Check sheet for the modelled part. Datum: model origin and axes. Units: mm. A direction names the side the tool comes from. Round coordinates to 2 decimals unless told otherwise and drop trailing zeros. Write each loop counter-clockwise with the first axis right and the second up, starting at its lowest first coordinate (ties: lowest second). Pieces come first, ordered by that corner, then holes. Notation, with made-up numbers: (68, 56) - (102, 56) arc R21 ccw to (102, 60) - close; hole circle Ø1 at (66, -12.5). An arc over 180 degrees is marked (long way). Use one line per item in the form item = value. Start each with the question number.
1) Scan lines: probe 1 along Z at (x, y) = (-1.5, -5); probe 2 along X at (y, z) = (-5.75, 16.5); probe 3 along Z at (x, y) = (5.25, 4.25). Record each from-to range of solid material in increasing order.
2) Gauge pin test, flat ends, axial feed: P1, Ø3, axis at y = 2, z = 31.5, coming from the +X side; P2, Ø1, axis at x = -4, y = 6, coming from the +Z side; P3, Ø8, axis at x = 0.5, y = 5.5, coming from the +Z side. Record the tip position at first contact, or that the pin passes through.
3) Section check C-C (z = 41). Record the boundary of the cut face in (x, y), then the cut area to 3 significant figures.
4) Section check B-B (z = 36). Record the boundary of the cut face in (x, y), then the cut area to 3 significant figures.
5) Set-up check for faces 1 (the face through (-3.746, 0.165, 37.708)), 2 (the face through (0, 0.75, 44)), 3 (the face through (0, -0.75, 44)): record each of +Z, -Z, +X, -X, +Y, -Y from which the full face is reachable in a straight line by a thin tool's end or side.
6) Section check A-A (z = 3). Record the boundary of the cut face in (x, y) (3 decimals).
from build123d import *

# Parameters (mm, degrees)
F1_DEPTH  = 20
F2_R      = 6
F3_DEPTH  = 15
F5_DEPTH  = 15
F6_COUNT  = 55
F8_R      = 3.75
F9_DEPTH  = 10
F11_DEPTH = 25


with BuildPart() as f1:
    # F0 (on Top) → F1 (new body)
    with BuildSketch(Plane.XY):
        Polygon((6.875, -3.969283), (6.875, 3.969283), (0, 7.938566), (-6.875, 3.969283), (-6.875, -3.969283), (0, -7.938566), align=None)
    extrude(amount=F1_DEPTH)

    # F2 (on face) → F3 (join)
    with BuildSketch(Plane.XY.offset(20)):
        Circle(F2_R)
    extrude(amount=F3_DEPTH)


with BuildPart() as f5:
    # F4 (on face) → F5 (new body, through all)
    with BuildSketch(Plane.XY.offset(35)):
        with BuildLine():
            ThreePointArc((0.365715, 5.988844), (0, 6), (-0.365715, 5.988844))
            Line((-0.365715, 5.988844), (0, 5.647886))
            Line((0, 5.647886), (0.365715, 5.988844))
        make_face()
    extrude(amount=-F5_DEPTH)


with BuildPart() as f6_1:
    # F6: instance of F5
    add(f5.part.rotate(Axis((0, 0, 35), (0, 0, -1)), 1 * 360 / F6_COUNT))


with BuildPart() as f6_2:
    # F6: instance of F5
    add(f5.part.rotate(Axis((0, 0, 35), (0, 0, -1)), 2 * 360 / F6_COUNT))


with BuildPart() as f6_3:
    # F6: instance of F5
    add(f5.part.rotate(Axis((0, 0, 35), (0, 0, -1)), 3 * 360 / F6_COUNT))


with BuildPart() as f6_4:
    # F6: instance of F5
    add(f5.part.rotate(Axis((0, 0, 35), (0, 0, -1)), 4 * 360 / F6_COUNT))


with BuildPart() as f6_5:
    # F6: instance of F5
    add(f5.part.rotate(Axis((0, 0, 35), (0, 0, -1)), 5 * 360 / F6_COUNT))


with BuildPart() as f6_6:
    # F6: instance of F5
    add(f5.part.rotate(Axis((0, 0, 35), (0, 0, -1)), 6 * 360 / F6_COUNT))


with BuildPart() as f6_7:
    # F6: instance of F5
    add(f5.part.rotate(Axis((0, 0, 35), (0, 0, -1)), 7 * 360 / F6_COUNT))


with BuildPart() as f6_8:
    # F6: instance of F5
    add(f5.part.rotate(Axis((0, 0, 35), (0, 0, -1)), 8 * 360 / F6_COUNT))


with BuildPart() as f6_9:
    # F6: instance of F5
    add(f5.part.rotate(Axis((0, 0, 35), (0, 0, -1)), 9 * 360 / F6_COUNT))


with BuildPart() as f6_10:
    # F6: instance of F5
    add(f5.part.rotate(Axis((0, 0, 35), (0, 0, -1)), 10 * 360 / F6_COUNT))


with BuildPart() as f6_11:
    # F6: instance of F5
    add(f5.part.rotate(Axis((0, 0, 35), (0, 0, -1)), 11 * 360 / F6_COUNT))


with BuildPart() as f6_12:
    # F6: instance of F5
    add(f5.part.rotate(Axis((0, 0, 35), (0, 0, -1)), 12 * 360 / F6_COUNT))


with BuildPart() as f6_13:
    # F6: instance of F5
    add(f5.part.rotate(Axis((0, 0, 35), (0, 0, -1)), 13 * 360 / F6_COUNT))


with BuildPart() as f6_14:
    # F6: instance of F5
    add(f5.part.rotate(Axis((0, 0, 35), (0, 0, -1)), 14 * 360 / F6_COUNT))


with BuildPart() as f6_15:
    # F6: instance of F5
    add(f5.part.rotate(Axis((0, 0, 35), (0, 0, -1)), 15 * 360 / F6_COUNT))


with BuildPart() as f6_16:
    # F6: instance of F5
    add(f5.part.rotate(Axis((0, 0, 35), (0, 0, -1)), 16 * 360 / F6_COUNT))


with BuildPart() as f6_17:
    # F6: instance of F5
    add(f5.part.rotate(Axis((0, 0, 35), (0, 0, -1)), 17 * 360 / F6_COUNT))


with BuildPart() as f6_18:
    # F6: instance of F5
    add(f5.part.rotate(Axis((0, 0, 35), (0, 0, -1)), 18 * 360 / F6_COUNT))


with BuildPart() as f6_19:
    # F6: instance of F5
    add(f5.part.rotate(Axis((0, 0, 35), (0, 0, -1)), 19 * 360 / F6_COUNT))


with BuildPart() as f6_20:
    # F6: instance of F5
    add(f5.part.rotate(Axis((0, 0, 35), (0, 0, -1)), 20 * 360 / F6_COUNT))


with BuildPart() as f6_21:
    # F6: instance of F5
    add(f5.part.rotate(Axis((0, 0, 35), (0, 0, -1)), 21 * 360 / F6_COUNT))


with BuildPart() as f6_22:
    # F6: instance of F5
    add(f5.part.rotate(Axis((0, 0, 35), (0, 0, -1)), 22 * 360 / F6_COUNT))


with BuildPart() as f6_23:
    # F6: instance of F5
    add(f5.part.rotate(Axis((0, 0, 35), (0, 0, -1)), 23 * 360 / F6_COUNT))


with BuildPart() as f6_24:
    # F6: instance of F5
    add(f5.part.rotate(Axis((0, 0, 35), (0, 0, -1)), 24 * 360 / F6_COUNT))


with BuildPart() as f6_25:
    # F6: instance of F5
    add(f5.part.rotate(Axis((0, 0, 35), (0, 0, -1)), 25 * 360 / F6_COUNT))


with BuildPart() as f6_26:
    # F6: instance of F5
    add(f5.part.rotate(Axis((0, 0, 35), (0, 0, -1)), 26 * 360 / F6_COUNT))


with BuildPart() as f6_27:
    # F6: instance of F5
    add(f5.part.rotate(Axis((0, 0, 35), (0, 0, -1)), 27 * 360 / F6_COUNT))


with BuildPart() as f6_28:
    # F6: instance of F5
    add(f5.part.rotate(Axis((0, 0, 35), (0, 0, -1)), 28 * 360 / F6_COUNT))


with BuildPart() as f6_29:
    # F6: instance of F5
    add(f5.part.rotate(Axis((0, 0, 35), (0, 0, -1)), 29 * 360 / F6_COUNT))


with BuildPart() as f6_30:
    # F6: instance of F5
    add(f5.part.rotate(Axis((0, 0, 35), (0, 0, -1)), 30 * 360 / F6_COUNT))


with BuildPart() as f6_31:
    # F6: instance of F5
    add(f5.part.rotate(Axis((0, 0, 35), (0, 0, -1)), 31 * 360 / F6_COUNT))


with BuildPart() as f6_32:
    # F6: instance of F5
    add(f5.part.rotate(Axis((0, 0, 35), (0, 0, -1)), 32 * 360 / F6_COUNT))


with BuildPart() as f6_33:
    # F6: instance of F5
    add(f5.part.rotate(Axis((0, 0, 35), (0, 0, -1)), 33 * 360 / F6_COUNT))


with BuildPart() as f6_34:
    # F6: instance of F5
    add(f5.part.rotate(Axis((0, 0, 35), (0, 0, -1)), 34 * 360 / F6_COUNT))


with BuildPart() as f6_35:
    # F6: instance of F5
    add(f5.part.rotate(Axis((0, 0, 35), (0, 0, -1)), 35 * 360 / F6_COUNT))


with BuildPart() as f6_36:
    # F6: instance of F5
    add(f5.part.rotate(Axis((0, 0, 35), (0, 0, -1)), 36 * 360 / F6_COUNT))


with BuildPart() as f6_37:
    # F6: instance of F5
    add(f5.part.rotate(Axis((0, 0, 35), (0, 0, -1)), 37 * 360 / F6_COUNT))


with BuildPart() as f6_38:
    # F6: instance of F5
    add(f5.part.rotate(Axis((0, 0, 35), (0, 0, -1)), 38 * 360 / F6_COUNT))


with BuildPart() as f6_39:
    # F6: instance of F5
    add(f5.part.rotate(Axis((0, 0, 35), (0, 0, -1)), 39 * 360 / F6_COUNT))


with BuildPart() as f6_40:
    # F6: instance of F5
    add(f5.part.rotate(Axis((0, 0, 35), (0, 0, -1)), 40 * 360 / F6_COUNT))


with BuildPart() as f6_41:
    # F6: instance of F5
    add(f5.part.rotate(Axis((0, 0, 35), (0, 0, -1)), 41 * 360 / F6_COUNT))


with BuildPart() as f6_42:
    # F6: instance of F5
    add(f5.part.rotate(Axis((0, 0, 35), (0, 0, -1)), 42 * 360 / F6_COUNT))


with BuildPart() as f6_43:
    # F6: instance of F5
    add(f5.part.rotate(Axis((0, 0, 35), (0, 0, -1)), 43 * 360 / F6_COUNT))


with BuildPart() as f6_44:
    # F6: instance of F5
    add(f5.part.rotate(Axis((0, 0, 35), (0, 0, -1)), 44 * 360 / F6_COUNT))


with BuildPart() as f6_45:
    # F6: instance of F5
    add(f5.part.rotate(Axis((0, 0, 35), (0, 0, -1)), 45 * 360 / F6_COUNT))


with BuildPart() as f6_46:
    # F6: instance of F5
    add(f5.part.rotate(Axis((0, 0, 35), (0, 0, -1)), 46 * 360 / F6_COUNT))


with BuildPart() as f6_47:
    # F6: instance of F5
    add(f5.part.rotate(Axis((0, 0, 35), (0, 0, -1)), 47 * 360 / F6_COUNT))


with BuildPart() as f6_48:
    # F6: instance of F5
    add(f5.part.rotate(Axis((0, 0, 35), (0, 0, -1)), 48 * 360 / F6_COUNT))


with BuildPart() as f6_49:
    # F6: instance of F5
    add(f5.part.rotate(Axis((0, 0, 35), (0, 0, -1)), 49 * 360 / F6_COUNT))


with BuildPart() as f6_50:
    # F6: instance of F5
    add(f5.part.rotate(Axis((0, 0, 35), (0, 0, -1)), 50 * 360 / F6_COUNT))


with BuildPart() as f6_51:
    # F6: instance of F5
    add(f5.part.rotate(Axis((0, 0, 35), (0, 0, -1)), 51 * 360 / F6_COUNT))


with BuildPart() as f6_52:
    # F6: instance of F5
    add(f5.part.rotate(Axis((0, 0, 35), (0, 0, -1)), 52 * 360 / F6_COUNT))


with BuildPart() as f6_53:
    # F6: instance of F5
    add(f5.part.rotate(Axis((0, 0, 35), (0, 0, -1)), 53 * 360 / F6_COUNT))


with BuildPart() as f6_54:
    # F6: instance of F5
    add(f5.part.rotate(Axis((0, 0, 35), (0, 0, -1)), 54 * 360 / F6_COUNT))


with BuildPart() as f1_1:
    add(f1.part)

    # F7: cut F6_6, F6_8, F6_10, F6_7, F6_1, F6_4, F6_5, F6_3, F6_2, F5, F6_9, F6_11, F6_12, F6_13, F6_14, F6_15, F6_16, F6_17, F6_18, F6_19, F6_20, F6_21, F6_22, F6_23, F6_24, F6_25, F6_26, F6_27, F6_28, F6_29, F6_30, F6_31, F6_32, F6_33, F6_34, F6_35, F6_36, F6_37, F6_38, F6_39, F6_40, F6_41, F6_42, F6_43, F6_44, F6_45, F6_46, F6_47, F6_48, F6_49, F6_50, F6_51, F6_52, F6_53, F6_54
    add(f6_6.part, mode=Mode.SUBTRACT)
    add(f6_8.part, mode=Mode.SUBTRACT)
    add(f6_10.part, mode=Mode.SUBTRACT)
    add(f6_7.part, mode=Mode.SUBTRACT)
    add(f6_1.part, mode=Mode.SUBTRACT)
    add(f6_4.part, mode=Mode.SUBTRACT)
    add(f6_5.part, mode=Mode.SUBTRACT)
    add(f6_3.part, mode=Mode.SUBTRACT)
    add(f6_2.part, mode=Mode.SUBTRACT)
    add(f5.part, mode=Mode.SUBTRACT)
    add(f6_9.part, mode=Mode.SUBTRACT)
    add(f6_11.part, mode=Mode.SUBTRACT)
    add(f6_12.part, mode=Mode.SUBTRACT)
    add(f6_13.part, mode=Mode.SUBTRACT)
    add(f6_14.part, mode=Mode.SUBTRACT)
    add(f6_15.part, mode=Mode.SUBTRACT)
    add(f6_16.part, mode=Mode.SUBTRACT)
    add(f6_17.part, mode=Mode.SUBTRACT)
    add(f6_18.part, mode=Mode.SUBTRACT)
    add(f6_19.part, mode=Mode.SUBTRACT)
    add(f6_20.part, mode=Mode.SUBTRACT)
    add(f6_21.part, mode=Mode.SUBTRACT)
    add(f6_22.part, mode=Mode.SUBTRACT)
    add(f6_23.part, mode=Mode.SUBTRACT)
    add(f6_24.part, mode=Mode.SUBTRACT)
    add(f6_25.part, mode=Mode.SUBTRACT)
    add(f6_26.part, mode=Mode.SUBTRACT)
    add(f6_27.part, mode=Mode.SUBTRACT)
    add(f6_28.part, mode=Mode.SUBTRACT)
    add(f6_29.part, mode=Mode.SUBTRACT)
    add(f6_30.part, mode=Mode.SUBTRACT)
    add(f6_31.part, mode=Mode.SUBTRACT)
    add(f6_32.part, mode=Mode.SUBTRACT)
    add(f6_33.part, mode=Mode.SUBTRACT)
    add(f6_34.part, mode=Mode.SUBTRACT)
    add(f6_35.part, mode=Mode.SUBTRACT)
    add(f6_36.part, mode=Mode.SUBTRACT)
    add(f6_37.part, mode=Mode.SUBTRACT)
    add(f6_38.part, mode=Mode.SUBTRACT)
    add(f6_39.part, mode=Mode.SUBTRACT)
    add(f6_40.part, mode=Mode.SUBTRACT)
    add(f6_41.part, mode=Mode.SUBTRACT)
    add(f6_42.part, mode=Mode.SUBTRACT)
    add(f6_43.part, mode=Mode.SUBTRACT)
    add(f6_44.part, mode=Mode.SUBTRACT)
    add(f6_45.part, mode=Mode.SUBTRACT)
    add(f6_46.part, mode=Mode.SUBTRACT)
    add(f6_47.part, mode=Mode.SUBTRACT)
    add(f6_48.part, mode=Mode.SUBTRACT)
    add(f6_49.part, mode=Mode.SUBTRACT)
    add(f6_50.part, mode=Mode.SUBTRACT)
    add(f6_51.part, mode=Mode.SUBTRACT)
    add(f6_52.part, mode=Mode.SUBTRACT)
    add(f6_53.part, mode=Mode.SUBTRACT)
    add(f6_54.part, mode=Mode.SUBTRACT)

    # F8 (on face) → F9 (join)
    with BuildSketch(Plane.XY.offset(35)):
        Circle(F8_R)
    extrude(amount=F9_DEPTH)

    # F10 (on face) → F11 (cut)
    with BuildSketch(Plane(origin=(-6.875, 0, 0), x_dir=(0, -1, 0), z_dir=(-1, 0, 0))):
        with BuildLine():
            Line((-0.75, 49.5), (-0.75, 50))
            Line((-0.75, 50), (-4.25, 50))
            Line((-4.25, 50), (-4.25, 36.5))
            ThreePointArc((-4.25, 36.5), (-1.673762, 39.586881), (-0.75, 43.5))
            Line((-0.75, 43.5), (-0.75, 49.5))
        make_face()
        with BuildLine():
            Line((0.75, 50), (0.75, 43.5))
            ThreePointArc((0.75, 43.5), (1.673762, 39.586881), (4.25, 36.5))
            Line((4.25, 36.5), (4.25, 50))
            Line((4.25, 50), (0.75, 50))
        make_face()
    extrude(amount=-F11_DEPTH, mode=Mode.SUBTRACT)


solid = f1_1.part
Results are:
q1.probe_1 = 0 to 35
q1.probe_2 = -3.79 to 3.79
q1.probe_3 = 0 to 20
q2.P1 = 5.91
q2.P2 = 20
q2.P3 = 39.96
q3.outline = (-3.58, -1.11) - (3.58, -1.11) arc R3.75 ccw to (3.58, 1.11) - (-3.58, 1.11) arc R3.75 ccw to start
q3.area = 16.5 mm²
q4.outline = circle Ø7.5 at (0, 0)
q4.area = 44.2 mm²
q5.face_1 = +Z
q5.face_2 = +Z, +X, -X, +Y
q5.face_3 = +Z, +X, -X, -Y
q6.outline = (-6.875, -3.969) - (0, -7.939) - (6.875, -3.969) - (6.875, 3.969) - (0, 7.939) - (-6.875, 3.969) - close
